from build123d import *

# Parameters (mm, degrees)
SKETCH1_W                = 80
SKETCH1_H                = 80
BOSS_EXTRUDE1_DEPTH      = 3.175
CUT_EXTRUDE3_START       = -3.175
CUT_EXTRUDE3_OUTLINE_W   = 3.175
CUT_EXTRUDE3_OUTLINE_H   = 5.333333334
CUT_EXTRUDE3_OUTLINE_H_2 = 5.333333333
CUT_EXTRUDE3_OUTLINE_W_2 = 5.333333334
CUT_EXTRUDE3_OUTLINE_H_3 = 3.175
CUT_EXTRUDE3_OUTLINE_W_3 = 5.333333333
CUT_EXTRUDE3_DEPTH       = 3.175
SKETCH3_W                = 80
SKETCH3_H                = 5.333333333
BOSS_EXTRUDE2_DEPTH      = 3.175


# Read off the part's stored shape, not the designer's step: Cut-Extrude3
with BuildPart() as part:
    # Sketch1 → Boss-Extrude1 (new body)
    with BuildSketch(Plane(origin=(0, 0, 0), x_dir=(1, 0, 0), z_dir=(0, 1, 0))):
        Rectangle(SKETCH1_W, SKETCH1_H)
    extrude(amount=BOSS_EXTRUDE1_DEPTH)

    # Cut-Extrude3 outline → Cut-Extrude3 (cut)
    with BuildSketch(Plane(origin=(0, 3.175, 0), x_dir=(1, 0, 0), z_dir=(0, 1, 0)).offset(CUT_EXTRUDE3_START)):
        with Locations((-38.4125, 32)):
            Rectangle(CUT_EXTRUDE3_OUTLINE_W, CUT_EXTRUDE3_OUTLINE_H)
        with Locations((-38.4125, 21.333333334)):
            Rectangle(CUT_EXTRUDE3_OUTLINE_W, CUT_EXTRUDE3_OUTLINE_H_2)
        with Locations((-32, 38.4125)):
            Rectangle(CUT_EXTRUDE3_OUTLINE_W_2, CUT_EXTRUDE3_OUTLINE_H_3)
        with Locations((-38.4125, 10.666666666)):
            Rectangle(CUT_EXTRUDE3_OUTLINE_W, CUT_EXTRUDE3_OUTLINE_H_2)
        with Locations((-21.333333334, 38.4125)):
            Rectangle(CUT_EXTRUDE3_OUTLINE_W_3, CUT_EXTRUDE3_OUTLINE_H_3)
        with Locations((-38.4125, 0)):
            Rectangle(CUT_EXTRUDE3_OUTLINE_W, CUT_EXTRUDE3_OUTLINE_H)
        with Locations((-10.666666666, 38.4125)):
            Rectangle(CUT_EXTRUDE3_OUTLINE_W_3, CUT_EXTRUDE3_OUTLINE_H_3)
        with Locations((-38.4125, -10.666666666)):
            Rectangle(CUT_EXTRUDE3_OUTLINE_W, CUT_EXTRUDE3_OUTLINE_H_2)
        with Locations((0, 38.4125)):
            Rectangle(CUT_EXTRUDE3_OUTLINE_W_2, CUT_EXTRUDE3_OUTLINE_H_3)
        with Locations((-38.4125, -21.333333334)):
            Rectangle(CUT_EXTRUDE3_OUTLINE_W, CUT_EXTRUDE3_OUTLINE_H_2)
        with Locations((10.666666666, 38.4125)):
            Rectangle(CUT_EXTRUDE3_OUTLINE_W_3, CUT_EXTRUDE3_OUTLINE_H_3)
        with Locations((-38.4125, -32)):
            Rectangle(CUT_EXTRUDE3_OUTLINE_W, CUT_EXTRUDE3_OUTLINE_H)
        with Locations((21.333333334, 38.4125)):
            Rectangle(CUT_EXTRUDE3_OUTLINE_W_3, CUT_EXTRUDE3_OUTLINE_H_3)
        with Locations((32, 38.4125)):
            Rectangle(CUT_EXTRUDE3_OUTLINE_W_2, CUT_EXTRUDE3_OUTLINE_H_3)
        with Locations((-32, -38.4125)):
            Rectangle(CUT_EXTRUDE3_OUTLINE_W_2, CUT_EXTRUDE3_OUTLINE_H_3)
        with Locations((-21.333333334, -38.4125)):
            Rectangle(CUT_EXTRUDE3_OUTLINE_W_3, CUT_EXTRUDE3_OUTLINE_H_3)
        with Locations((38.4125, 32)):
            Rectangle(CUT_EXTRUDE3_OUTLINE_W, CUT_EXTRUDE3_OUTLINE_H)
        with Locations((-10.666666666, -38.4125)):
            Rectangle(CUT_EXTRUDE3_OUTLINE_W_3, CUT_EXTRUDE3_OUTLINE_H_3)
        with Locations((38.4125, 21.333333334)):
            Rectangle(CUT_EXTRUDE3_OUTLINE_W, CUT_EXTRUDE3_OUTLINE_H_2)
        with Locations((0, -38.4125)):
            Rectangle(CUT_EXTRUDE3_OUTLINE_W_2, CUT_EXTRUDE3_OUTLINE_H_3)
        with Locations((38.4125, 10.666666666)):
            Rectangle(CUT_EXTRUDE3_OUTLINE_W, CUT_EXTRUDE3_OUTLINE_H_2)
        with Locations((10.666666666, -38.4125)):
            Rectangle(CUT_EXTRUDE3_OUTLINE_W_3, CUT_EXTRUDE3_OUTLINE_H_3)
        with Locations((38.4125, 0)):
            Rectangle(CUT_EXTRUDE3_OUTLINE_W, CUT_EXTRUDE3_OUTLINE_H)
        with Locations((21.333333334, -38.4125)):
            Rectangle(CUT_EXTRUDE3_OUTLINE_W_3, CUT_EXTRUDE3_OUTLINE_H_3)
        with Locations((38.4125, -10.666666666)):
            Rectangle(CUT_EXTRUDE3_OUTLINE_W, CUT_EXTRUDE3_OUTLINE_H_2)
        with Locations((32, -38.4125)):
            Rectangle(CUT_EXTRUDE3_OUTLINE_W_2, CUT_EXTRUDE3_OUTLINE_H_3)
        with Locations((38.4125, -21.333333334)):
            Rectangle(CUT_EXTRUDE3_OUTLINE_W, CUT_EXTRUDE3_OUTLINE_H_2)
        with Locations((38.4125, -32)):
            Rectangle(CUT_EXTRUDE3_OUTLINE_W, CUT_EXTRUDE3_OUTLINE_H)
    extrude(amount=CUT_EXTRUDE3_DEPTH, mode=Mode.SUBTRACT)

    # Sketch3 → Boss-Extrude2 (add)
    with BuildSketch(Plane.XZ):
        with Locations((0, 37.333333334)):
            Rectangle(SKETCH3_W, SKETCH3_H)
    extrude(amount=-BOSS_EXTRUDE2_DEPTH)


solid = part.part
The listing builds one solid part. Answer for the finished solid, in the listing's coordinates (mm). A direction names the side the tool comes from. Round coordinates to 2 decimals unless told otherwise and drop trailing zeros. Write each loop counter-clockwise with the first axis right and the second up, starting at its lowest first coordinate (ties: lowest second). Pieces come first, ordered by that corner, then holes. Notation, with made-up numbers: (-11.5, 64) - (-7.5, 64) arc R34 cw to (-7.5, 101) - close; hole circle Ø5 at (56.25, -12). An arc over 180 degrees is marked (long way). Use a Markdown table: item, result. Add a question column.
1. The part is cut by section A-A (z = -10). Write down the section's boundary in (x, y) (3 decimals), and give its area (3 significant figures).
2. The part is cut by section B-B (x = 20.5). Write down the section's boundary in (y, z) (3 decimals), and give its area (3 significant figures).
3. A tool of negligible diameter and unlimited length cuts with its end or side. For faces 4 (the face through (13.333, 2, -38)), 5 (the face through (-40, 2, -5)), 6 (the face through (-38, 2, 2.667)), 7 (the face through (36.825, 2, -21)), from which of +Z, -Z, +X, -X, +Y, -Y can it reach the whole face along a straight path? Write none if from no direction.
4. A flat-ended cylindrical pin translates along its axis: P1, Ø1, axis at x = 22, y = 2, coming from the -Z side (3 decimals). Find the tip coordinate at first contact, or state that the pin passes through.
5. Consider line 1 (Z direction, x = -19.5, y = 1.2) (3 decimals); line 2 (X direction, y = 2.3, z = -19.5) (3 decimals). Determine where each line is inside the solid, lowest interval first.
6. For a pull along Z with two mould halves and no side action, classify faces 1 (the face through (36.825, 2, 21)), 2 (the face through (-32, 2, -36.825)), 3 (the face through (-40, 2, -37)) as +Z half, -Z half, draft (parallel to the pull), parting line (faces both ways), or undercut.
Reported:
| question | item | result |
|---|---|---|
| 1 | outline | (-36.825, 0) - (36.825, 0) - (36.825, 3.175) - (-36.825, 3.175) - close |
| 1 | area | 234 mm^2 |
| 2 | outline | (0, -36.825) - (3.175, -36.825) - (3.175, 40) - (0, 40) - close |
| 2 | area | 244 mm^2 |
| 3 | face 4 | -Z, +Y, -Y |
| 3 | face 5 | +Z, -Z, -X, +Y, -Y |
| 3 | face 6 | -X, +Y, -Y |
| 3 | face 7 | +X, +Y, -Y |
| 4 | P1 | z = -36.825 |
| 5 | line 1 | -36.825 to 40 |
| 5 | line 2 | -36.825 to 36.825 |
| 6 | face 1 | undercut |
| 6 | face 2 | -Z half |
| 6 | face 3 | draft |
